Input: part model. Units: mm. Frame: model coordinates. A direction names the side the tool comes from. Round coordinates to 2 decimals unless told otherwise and drop trailing zeros. Loops run counter-clockwise (first coordinate to the right, second up) from the corner with the lowest first, then second, coordinate; pieces in that order, holes last.
1) Section B-B, the plane y = 16. Return loops of the section in (x, z), and give its area (3 significant figures).
2) Draft query along X for faces 1 (the face through (8, 12.5, 2)), 2 (the face through (0, 12.5, 2)), 3 (the face through (11, 22, 2)). Return one class per face: pulls with the +X half, pulls with the -X half, needs draft (parallel to the pull), parting line crosses it, or undercut.
3) Section D-D, the plane x = 1. Return loops of the section in (y, z), and give its area (4 significant figures).
4) Access query for faces 4 (the face through (-8, 12.5, 2)), 5 (the face through (-3.993, -12.863, 2.465)), 6 (the face through (6, 32.5, 2)). Directions: +Z, -Z, +X, -X, +Y, -Y. A direction counts if a zero-diameter tool reaches every point of the face in a straight line with its end or side. Return the directions, or none.
5) Section A-A, the plane x = -6. Return loops of the section in (y, z), and give its area (3 significant figures).
6) First-contact query: pin 1 (1 mm diameter, centred on x = 0, z = 0.5, fed in from -Y); pin 2 (1.6 mm diameter, centred on y = 31.5, z = 2.5, fed in from +X); pin 3 (1.5 mm diameter, centred on y = 0.5, z = 2, fed in from -X). Flat tips, straight axial feed; report the tip coordinate or a pass-through.
7) Ray query, line 1 along X through (y, z) = (3, 3.55); line 2 along X through (y, z) = (22.5, 2.6); line 3 along Y through (x, z) = (7, 1.45). Return the intervals inside material, ascending.
from build123d import *

# Parameters (mm, degrees)
F1_DEPTH = 5


with BuildPart() as f1:
    # F0 (on Top) → F1 (new body)
    with BuildSketch(Plane.XY):
        with BuildLine():
            Line((-4.5, 12.5), (0, 12.5))
            Line((0, 12.5), (4.5, 12.5))
            Line((4.5, 12.5), (4.5, 0))
            Line((4.5, 0), (4.5, -11.917724))
            Line((4.5, -11.917724), (3.5, -13.781429))
            Line((3.5, -13.781429), (3.5, -14.5))
            Line((3.5, -14.5), (6.5, -14.5))
            Line((6.5, -14.5), (6.5, -12.5))
            Line((6.5, -12.5), (6.5, 12.5))
            Line((6.5, 12.5), (9, 12.5))
            ThreePointArc((9, 12.5), (10.414214, 13.085786), (11, 14.5))
            Line((11, 14.5), (11, 30.5))
            ThreePointArc((11, 30.5), (10.414214, 31.914214), (9, 32.5))
            Line((9, 32.5), (2, 32.5))
            Line((2, 32.5), (2, 30.5))
            Line((2, 30.5), (7, 30.5))
            ThreePointArc((7, 30.5), (8.414214, 29.914214), (9, 28.5))
            Line((9, 28.5), (9, 14.5))
            Line((9, 14.5), (-9, 14.5))
            Line((-9, 14.5), (-9, 28.5))
            ThreePointArc((-9, 28.5), (-8.414214, 29.914214), (-7, 30.5))
            Line((-7, 30.5), (-2, 30.5))
            Line((-2, 30.5), (-2, 32.5))
            Line((-2, 32.5), (-9, 32.5))
            ThreePointArc((-9, 32.5), (-10.414214, 31.914214), (-11, 30.5))
            Line((-11, 30.5), (-11, 14.5))
            ThreePointArc((-11, 14.5), (-10.414214, 13.085786), (-9, 12.5))
            Line((-9, 12.5), (-6.5, 12.5))
            Line((-6.5, 12.5), (-6.5, -12.5))
            Line((-6.5, -12.5), (-6.5, -14.5))
            Line((-6.5, -14.5), (-3.5, -14.5))
            Line((-3.5, -14.5), (-3.5, -13.781429))
            Line((-3.5, -13.781429), (-4.5, -11.917724))
            Line((-4.5, -11.917724), (-4.5, 12.5))
        make_face()
    extrude(amount=F1_DEPTH)


solid = f1.part
Final values:
1. outline: (-11, 0) - (-9, 0) - (-9, 5) - (-11, 5) - close; (9, 0) - (11, 0) - (11, 5) - (9, 5) - close
1. area: 20.0 mm2
2. face 1: needs draft
2. face 2: undercut
2. face 3: pulls with the +X half
3. outline: (12.5, 0) - (14.5, 0) - (14.5, 5) - (12.5, 5) - close
3. area: 10.00 mm2
4. face 4: +Z, -Z, -X, -Y
4. face 5: +Z, -Z
4. face 6: +Z, -Z, +X, -X, +Y
5. outline: (-14.5, 0) - (14.5, 0) - (14.5, 5) - (-14.5, 5) - close; (30.5, 0) - (32.5, 0) - (32.5, 5) - (30.5, 5) - close
5. area: 155 mm2
6. pin 1: stops at y = 12.5
6. pin 2: stops at x = 10.99
6. pin 3: stops at x = -6.5
7. line 1: x = -6.5 to -4.5, 4.5 to 6.5
7. line 2: x = -11 to -9, 9 to 11
7. line 3: y = 12.5 to 14.5, 30.5 to 32.5
